Design review of the part built by this model. Coordinates are the model's own, in mm. A direction names the side the tool comes from. Give positions to 0.01 mm unless a question says otherwise; leave off trailing zeros. Loops run counter-clockwise (first coordinate to the right, second up) from the corner with the lowest first, then second, coordinate; pieces in that order, holes last. Notation, with made-up numbers: (48.25, 8) - (74.25, 8) arc R14 cw to (74.25, 27) - close; hole circle Ø7 at (89, 81.25). An arc over 180 degrees is marked (long way). Write each question's results on one line, items separated by ' | '.
from build123d import *

# Parameters (mm, degrees)
SKETCH1_W           = 35
SKETCH1_H           = 60
BOSS_EXTRUDE1_DEPTH = 2.5
SKETCH2_R           = 1
CUT_EXTRUDE1_DEPTH  = 5
FILLET1_R           = 15
SKETCH3_W           = 50
SKETCH3_H           = 5
BOSS_EXTRUDE2_DEPTH = 80
BOSS_EXTRUDE3_DEPTH = 2.5
SKETCH5_W           = 50
SKETCH5_H           = 5
BOSS_EXTRUDE4_DEPTH = 40
BOSS_EXTRUDE5_DEPTH = 1.5


with BuildPart() as part:
    # Sketch1 → Boss-Extrude1 (new, symmetric)
    with BuildSketch(Plane.XY):
        Rectangle(SKETCH1_W, SKETCH1_H)
    extrude(amount=BOSS_EXTRUDE1_DEPTH, both=True)

    # Sketch2 → Cut-Extrude1 (cut)
    with BuildSketch(Plane(origin=(0, 0, -2.5), x_dir=(-1, 0, 0), z_dir=(0, 0, -1))):
        with Locations((0, 25)):
            Circle(SKETCH2_R)
        with Locations((0, 22)):
            Circle(SKETCH2_R)
        with Locations((0, 19)):
            Circle(SKETCH2_R)
        with Locations((11.691342951, 18.25)):
            Circle(SKETCH2_R)
        with Locations((9.09326674, 16.75)):
            Circle(SKETCH2_R)
        with Locations((6.495190528, 15.25)):
            Circle(SKETCH2_R)
        with Locations((11.691342951, 4.75)):
            Circle(SKETCH2_R)
        with Locations((9.09326674, 6.25)):
            Circle(SKETCH2_R)
        with Locations((6.495190528, 7.75)):
            Circle(SKETCH2_R)
        with Locations((0, -2)):
            Circle(SKETCH2_R)
        with Locations((0, 1)):
            Circle(SKETCH2_R)
        with Locations((0, 4)):
            Circle(SKETCH2_R)
        with Locations((-11.691342951, 4.75)):
            Circle(SKETCH2_R)
        with Locations((-9.09326674, 6.25)):
            Circle(SKETCH2_R)
        with Locations((-6.495190528, 7.75)):
            Circle(SKETCH2_R)
        with Locations((-11.691342951, 18.25)):
            Circle(SKETCH2_R)
        with Locations((-9.09326674, 16.75)):
            Circle(SKETCH2_R)
        with Locations((-6.495190528, 15.25)):
            Circle(SKETCH2_R)
    extrude(amount=-CUT_EXTRUDE1_DEPTH, mode=Mode.SUBTRACT)

    # Fillet1
    fillet1_edges = [part.edges().sort_by_distance(p)[0] for p in [
        (-17.5, 30, 0),
        (17.5, 30, 0),
    ]]
    fillet(fillet1_edges, radius=FILLET1_R)

    # Sketch3 → Boss-Extrude2 (add)
    with BuildSketch(Plane(origin=(0, 0, -2.5), x_dir=(-1, 0, 0), z_dir=(0, 0, -1))):
        with Locations((0, -32.5)):
            Rectangle(SKETCH3_W, SKETCH3_H)
    extrude(amount=-BOSS_EXTRUDE2_DEPTH)

    # Sketch4 → Boss-Extrude3 (add, symmetric)
    with BuildSketch(Plane(origin=(0, 0, 0), x_dir=(0, 0, -1), z_dir=(1, 0, 0))):
        Polygon((-12.5, -30), (-2.5, -30), (-2.5, -15), align=None)
    extrude(amount=BOSS_EXTRUDE3_DEPTH, both=True)

    # Sketch5 → Boss-Extrude4 (add)
    with BuildSketch(Plane(origin=(0, 0, -2.5), x_dir=(-1, 0, 0), z_dir=(0, 0, -1))):
        with Locations((0, -32.5)):
            Rectangle(SKETCH5_W, SKETCH5_H)
    extrude(amount=BOSS_EXTRUDE4_DEPTH)

    # Sketch6 → Boss-Extrude5 (add, symmetric)
    with BuildSketch(Plane(origin=(0, 0, 0), x_dir=(0, 0, -1), z_dir=(1, 0, 0))):
        Polygon((2.5, -30), (8.5, -30), (2.5, -20), align=None)
    extrude(amount=BOSS_EXTRUDE5_DEPTH, both=True)


solid = part.part
(1) Take a section at B-B on y = -23. Give the boundary of the cut face in (x, z).
Answers below:
outline: (-17.5, -2.5) - (-1.5, -2.5) - (-1.5, -4.3) - (1.5, -4.3) - (1.5, -2.5) - (17.5, -2.5) - (17.5, 2.5) - (2.5, 2.5) - (2.5, 7.83) - (-2.5, 7.83) - (-2.5, 2.5) - (-17.5, 2.5) - close
(2) Wall thickness on line 1 along Z through (x, y) = (17, 5.5); line 2 along Y through (x, z) = (-0.5, 44): over which ranges is each line inside the solid? List them lowest first. Write a range as from..to.
Answers below:
line 1: -2.5..2.5 | line 2: -35..-30
(3) Take a section at A-A on z = 4. Give the boundary of the cut face in (x, y), plus the area to 3 significant figures.
Answers below:
outline: (-25, -35) - (25, -35) - (25, -30) - (2.5, -30) - (2.5, -17.25) - (-2.5, -17.25) - (-2.5, -30) - (-25, -30) - close | area: 314 mm2
(4) Insertion check: P1, Ø5.5, axis at y = -9, z = -0.5, coming from the +X side; P2, Ø5, axis at x = -19, y = -17.5, coming from the -Z side; P3, Ø2.5, axis at x = -6.5, y = 15.25, coming from the +Z side; P4, Ø11, axis at y = -25, z = 7.5, coming from the +X side. Each pin has a flat end and moves straight along its axis. Give the tip position at first contact, or say it passes through.
Answers below:
P1: x = 17.5 | P2: z = -2.5 | P3: z = 2.5 | P4: x = 25
(5) Tool access review of faces 1 (the flat face through (17.5, -8, 0)), 2 (the flat face through (-17.5, -8, 0)), 3 (the flat face through (-2.5, -26, 5)): name each direction out of +Z, -Z, +X, -X, +Y, -Y from which nothing blocks a thin tool from reaching the whole face with its end or side.
Answers below:
face 1: +Z, -Z, +X, +Y | face 2: +Z, -Z, -X, +Y | face 3: +Z, -X, +Y
(6) Take a section at C-C on z = 51.5. Give the boundary of the cut face in (x, y), plus the area to 3 significant figures.
Answers below:
outline: (-25, -35) - (25, -35) - (25, -30) - (-25, -30) - close | area: 250 mm2
(7) Take a section at D-D on y = 10.5. Give the boundary of the cut face in (x, z), plus the area to 3 significant figures.
Answers below:
outline: (-17.5, -2.5) - (17.5, -2.5) - (17.5, 2.5) - (-17.5, 2.5) - close | area: 175 mm2
(8) Draft analysis for pull direction Z (two halves, no side actions). For faces 4 (the flat face through (0, -32, 77.5)), 5 (the flat face through (0, -30, 18)), 6 (the flat face through (4, 0, -2.5)), state which applies: pulls with the +Z half, pulls with the -Z half, needs draft (parallel to the pull), parting line crosses it, or undercut.
Answers below:
face 4: pulls with the +Z half | face 5: needs draft | face 6: pulls with the -Z half
